Here's how the part is built. I have some questions about the finished solid (model axes, mm). Face numbers are marked on the shaded views. Coordinates: 2 decimals unless noted, no trailing zeros. Loops run counter-clockwise (first coordinate to the right, second up) from the corner with the lowest first, then second, coordinate; pieces in that order, holes last. Notation, with made-up numbers: (77.25, -3.5) -> (127.25, -3.5) arc R19 cw to (127.25, 28.5) -> close; hole circle Ø7 at (35.5, 56). An arc over 180 degrees is marked (long way). Answer as a JSON object with one key per item and string values. Group by question number.
1) I want a section at C-C (z = 15). Write out the boundary of the cut face in (x, y), then the cut area to 3 significant figures.
2) If we mould it in two halves opening along Z, with no side actions, what happens to the marked faces 1, 2 and 3? For each: +Z half, -Z half, draft (parallel to the pull), parting line (faces both ways), or undercut.
3) I need wall thicknesses on probe 1 along X at (y, z) = (20.5, 7.5); probe 2 along Z at (x, y) = (7.5, 24); probe 3 along Z at (x, y) = (7, 18.5). Which ranges of each line are inside material? Lowest first, please. Write a range as [from, to].
4) I want a section at A-A (y = 22). Write out the boundary of the cut face in (x, z).
5) I want a section at B-B (x = 14.25). Write out the boundary of the cut face in (y, z).
6) I want a section at D-D (y = 27). Write out the boundary of the cut face in (x, z), then the cut area to 3 significant figures.
Autodesk Inventor part; units mm, degrees
ref_plane "YZ Plane" through (0, 0, 0) normal (1, 0, 0) x (0, 1, 0)
ref_plane "XZ Plane" through (0, 0, 0) normal (0, 1, 0) x (-1, 0, 0)
ref_plane "XY Plane" through (0, 0, 0) normal (0, 0, 1) x (1, 0, 0)
sketch "Sketch1" plane through (0, 0, 0) normal (0, 0, 1) x (1, 0, 0)
  line L0 (0, 0) -> (15, 0)
  line L1 (15, 0) -> (15, 30)
  line L2 (15, 30) -> (0, 30)
  line L3 (0, 30) -> (0, 0)
  dimension "d0" = 30
  dimension "d1" = 15
extrude "Extrusion1" add sketch "Sketch1" along normal blind 17
sketch "Sketch2" plane through (15, 0, 0) normal (1, 0, 0) x (0, 0, -1)
  line L0 (-17, 0) -> (-17, 30)
  line L1 (-17, 30) -> (-6.0809, 0)
  line L2 (-17, 30) -> (14.9253, 30) construction
  line L3 (-6.0809, 0) -> (-17, 0)
  line L4 (-6.0809, 0) -> (-17, 0)
  line L5 (-17, 30) -> (-17, 0)
  dimension "d4" = 70
extrude "Extrusion2" cut sketch "Sketch2" against normal through all
sketch "Sketch3" plane through (0, 30, 0) normal (0, 1, 0) x (1, 0, 0)
  circle A0 centre (7.5, -7.5) radius 3.9624
  line L0 (15, -17) -> (0, -17) construction
  line L1 (7.5, -17) -> (7.5, 2) construction
  line L2 (0, 0) -> (0, -17) construction
  line L3 (0, -8.5) -> (15, -8.5) construction
  dimension "d7" = 7.9248
hole "Hole1" at (7.5, 30, 7.5) direction (0, -1, 0) diameter 7.9248 depth 12.7 tip angle 118
properties part number "Halter"
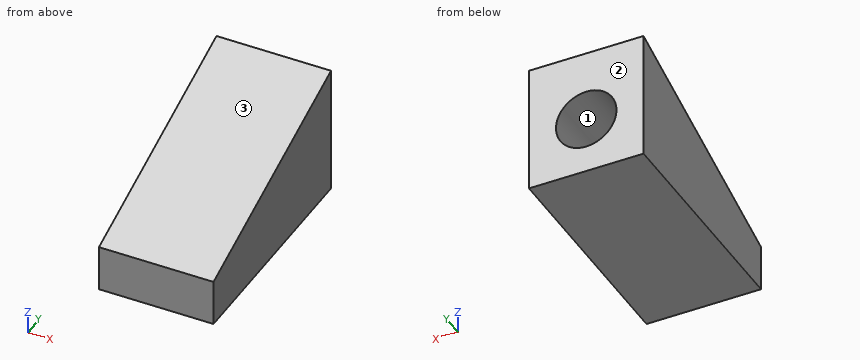
Determined:
{
 "1": {"outline": "(0, 24.51) -> (15, 24.51) -> (15, 30) -> (0, 30) -> close", "area": "82.4 mm^2"},
 "2": {"face 1": "undercut", "face 2": "draft", "face 3": "+Z half"},
 "3": {"probe 1": "[0, 3.54], [11.46, 15]", "probe 2": "[0, 3.54], [11.46, 14.82]", "probe 3": "[0, 3.57], [11.43, 12.81]"},
 "4": {"outline": "(0, 0) -> (15, 0) -> (15, 14.09) -> (0, 14.09) -> close; hole circle Ø7.92 at (7.5, 7.5)"},
 "5": {"outline": "(0, 0) -> (30, 0) -> (30, 17) -> (0, 6.08) -> close"},
 "6": {"outline": "(0, 0) -> (15, 0) -> (15, 15.91) -> (0, 15.91) -> close; hole circle Ø7.92 at (7.5, 7.5)", "area": "189 mm^2"}
}
